```python
from build123d import *

# Parameters (mm, degrees)
SKETCH1_W           = 100
SKETCH1_H           = 100
BOSS_EXTRUDE1_DEPTH = 100
CUT_EXTRUDE16_DEPTH = 70
SKETCH8_W           = 70
SKETCH8_H           = 70
CUT_EXTRUDE17_DEPTH = 30
SKETCH9_W           = 21
SKETCH9_H           = 21
CUT_EXTRUDE20_DEPTH = 90
SKETCH10_W          = 30
SKETCH10_H          = 30
SKETCH10_W_2        = 16
SKETCH10_H_2        = 16
CUT_EXTRUDE21_DEPTH = 50
SKETCH11_W          = 30
SKETCH11_H          = 30
SKETCH11_W_2        = 20
SKETCH11_H_2        = 20
CUT_EXTRUDE22_DEPTH = 20
SKETCH12_W          = 30
SKETCH12_H          = 30
SKETCH12_W_2        = 20
SKETCH12_H_2        = 20
CUT_EXTRUDE23_DEPTH = 70
SKETCH13_W          = 20
SKETCH13_H          = 20
SKETCH13_W_2        = 16
SKETCH13_H_2        = 16
CUT_EXTRUDE24_DEPTH = 50
SKETCH15_R          = 2
CUT_EXTRUDE25_DEPTH = 30
SKETCH16_R          = 2
CUT_EXTRUDE26_DEPTH = 30
SKETCH17_R          = 2
CUT_EXTRUDE27_DEPTH = 16
SKETCH18_R          = 2
CUT_EXTRUDE29_DEPTH = 16
SKETCH19_W          = 30
SKETCH19_H          = 30
CUT_EXTRUDE30_DEPTH = 5
BOSS_EXTRUDE2_DEPTH = 20
SKETCH21_W          = 20
SKETCH21_H          = 7
BOSS_EXTRUDE6_DEPTH = 24
SKETCH22_W          = 2.5
SKETCH22_H          = 2.5
CUT_EXTRUDE31_DEPTH = 20
SKETCH23_W          = 7
SKETCH23_H          = 20
BOSS_EXTRUDE7_DEPTH = 24


with BuildPart() as part:
    # Sketch1 → Boss-Extrude1 (new body)
    with BuildSketch(Plane.XY):
        Rectangle(SKETCH1_W, SKETCH1_H)
    extrude(amount=-BOSS_EXTRUDE1_DEPTH)

    # Sketch5 → Cut-Extrude16 (cut)
    with BuildSketch(Plane(origin=(0, 0, -100), x_dir=(-1, 0, 0), z_dir=(0, 0, -1))):
        Polygon((50, -50), (50, 50), (-50, 50), (-50, -20), (-20, -20), (-20, -50), align=None)
    extrude(amount=-CUT_EXTRUDE16_DEPTH, mode=Mode.SUBTRACT)

    # Sketch8 → Cut-Extrude17 (cut)
    with BuildSketch(Plane(origin=(0, 0, -30), x_dir=(-1, 0, 0), z_dir=(0, 0, -1))):
        with Locations((15, 15)):
            Rectangle(SKETCH8_W, SKETCH8_H)
    extrude(amount=-CUT_EXTRUDE17_DEPTH, mode=Mode.SUBTRACT)

    # Sketch9 → Cut-Extrude20 (cut)
    with BuildSketch(Plane(origin=(0, 0, -100), x_dir=(-1, 0, 0), z_dir=(0, 0, -1))):
        with Locations((-35, -35)):
            Rectangle(SKETCH9_W, SKETCH9_H)
    extrude(amount=-CUT_EXTRUDE20_DEPTH, mode=Mode.SUBTRACT)

    # Sketch10 → Cut-Extrude21 (cut)
    with BuildSketch(Plane.ZY.offset(50)):
        with Locations((-15, -35)):
            Rectangle(SKETCH10_W, SKETCH10_H)
        with Locations((-15, -35)):
            Rectangle(SKETCH10_W_2, SKETCH10_H_2, mode=Mode.SUBTRACT)
    extrude(amount=-CUT_EXTRUDE21_DEPTH, mode=Mode.SUBTRACT)

    # Sketch11 → Cut-Extrude22 (cut)
    with BuildSketch(Plane.ZY):
        with Locations((-15, -35)):
            Rectangle(SKETCH11_W, SKETCH11_H)
        with Locations((-15, -35)):
            Rectangle(SKETCH11_W_2, SKETCH11_H_2, mode=Mode.SUBTRACT)
    extrude(amount=-CUT_EXTRUDE22_DEPTH, mode=Mode.SUBTRACT)

    # Sketch12 → Cut-Extrude23 (cut)
    with BuildSketch(Plane(origin=(0, 50, 0), x_dir=(1, 0, 0), z_dir=(0, 1, 0))):
        with Locations((35, 15)):
            Rectangle(SKETCH12_W, SKETCH12_H)
        with Locations((35, 15)):
            Rectangle(SKETCH12_W_2, SKETCH12_H_2, mode=Mode.SUBTRACT)
    extrude(amount=-CUT_EXTRUDE23_DEPTH, mode=Mode.SUBTRACT)

    # Sketch13 → Cut-Extrude24 (cut)
    with BuildSketch(Plane(origin=(0, 50, 0), x_dir=(1, 0, 0), z_dir=(0, 1, 0))):
        with Locations((35, 15)):
            Rectangle(SKETCH13_W, SKETCH13_H)
        with Locations((35, 15)):
            Rectangle(SKETCH13_W_2, SKETCH13_H_2, mode=Mode.SUBTRACT)
    extrude(amount=-CUT_EXTRUDE24_DEPTH, mode=Mode.SUBTRACT)

    # Sketch15 → Cut-Extrude25 (cut)
    with BuildSketch(Plane(origin=(0, -20, 0), x_dir=(1, 0, 0), z_dir=(0, 1, 0))):
        with Locations(Location((35, 85, 0), (0, 0, 270))):
            Circle(SKETCH15_R)
        with Locations(Location((35, 45, 0), (0, 0, 270))):
            Circle(SKETCH15_R)
    extrude(amount=-CUT_EXTRUDE25_DEPTH, mode=Mode.SUBTRACT)

    # Sketch16 → Cut-Extrude26 (cut)
    with BuildSketch(Plane(origin=(50, 0, 0), x_dir=(0, 0, -1), z_dir=(1, 0, 0))):
        with Locations((75, -35)):
            Circle(SKETCH16_R)
        with Locations((35, -35)):
            Circle(SKETCH16_R)
    extrude(amount=-CUT_EXTRUDE26_DEPTH, mode=Mode.SUBTRACT)

    # Sketch17 → Cut-Extrude27 (cut)
    with BuildSketch(Plane(origin=(0, 0, -23), x_dir=(-1, 0, 0), z_dir=(0, 0, -1))):
        with Locations((-35, 30)):
            Circle(SKETCH17_R)
        with Locations((-35, 10)):
            Circle(SKETCH17_R)
    extrude(amount=-CUT_EXTRUDE27_DEPTH, mode=Mode.SUBTRACT)

    # Sketch18 → Cut-Extrude29 (cut)
    with BuildSketch(Plane(origin=(0, 0, -23), x_dir=(-1, 0, 0), z_dir=(0, 0, -1))):
        with Locations((30, -35)):
            Circle(SKETCH18_R)
        with Locations((10, -35)):
            Circle(SKETCH18_R)
    extrude(amount=-CUT_EXTRUDE29_DEPTH, mode=Mode.SUBTRACT)

    # Sketch19 → Cut-Extrude30 (cut)
    with BuildSketch(Plane.XY):
        with Locations((35, -35)):
            Rectangle(SKETCH19_W, SKETCH19_H)
    extrude(amount=-CUT_EXTRUDE30_DEPTH, mode=Mode.SUBTRACT)

    # Sketch20 → Boss-Extrude2 (add)
    with BuildSketch(Plane.XY.offset(-5)):
        Polygon((25, 0), (0, -25), (0, -27), (27, -27), (27, 0), align=None)
    extrude(amount=-BOSS_EXTRUDE2_DEPTH)

    # Sketch21 → Boss-Extrude6 (add)
    with BuildSketch(Plane.ZY):
        with Locations((-15, -46.5)):
            Rectangle(SKETCH21_W, SKETCH21_H)
    extrude(amount=-BOSS_EXTRUDE6_DEPTH)

    # Sketch22 → Cut-Extrude31 (cut)
    with BuildSketch(Plane(origin=(0, 0, -25), x_dir=(-1, 0, 0), z_dir=(0, 0, -1))):
        with Locations((-25.75, -25.75)):
            Rectangle(SKETCH22_W, SKETCH22_H)
    extrude(amount=-CUT_EXTRUDE31_DEPTH, mode=Mode.SUBTRACT)

    # Sketch23 → Boss-Extrude7 (add)
    with BuildSketch(Plane(origin=(0, 0, 0), x_dir=(1, 0, 0), z_dir=(0, 1, 0))):
        with Locations((46.5, 15)):
            Rectangle(SKETCH23_W, SKETCH23_H)
    extrude(amount=-BOSS_EXTRUDE7_DEPTH)


solid = part.part
```
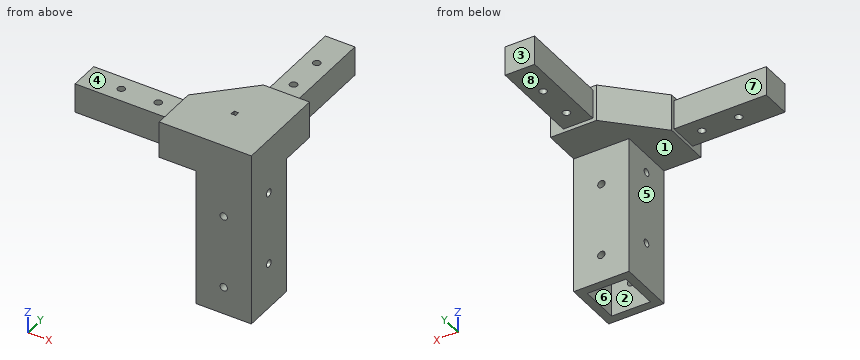
Verification items for the finished model (mm, model axes). Face numbers are marked on the shaded views. A direction names the side the tool comes from. Coordinates: 2 decimals unless noted, no trailing zeros. Order: outer loops, then holes, each group sorted by start corner. A loop starts at its lowest first (then second) coordinate and runs counter-clockwise, first axis right, second up. Notation, with made-up numbers: (33.25, 68.25) -> (71.25, 68.25) arc R33 ccw to (71.25, 100.25) -> close; hole circle Ø9 at (-8, -39.75). An arc over 180 degrees is marked (long way). Answer as CSV lines item,"result". Start each with the question number.
1) Cross-section at D-D, the plane x = -30. Record the boundary of the cut face in (y, z).
2) Set-up check for the marked faces 4, 5, 6, 7 and 8: record each of +Z, -Z, +X, -X, +Y, -Y from which the full face is reachable in a straight line by a thin tool's end or side.
3) Gauge pin test, flat ends, axial feed: pin 1 Ø13 at (y, z) = (13, -17.5) entering from -X; pin 2 Ø17 at (y, z) = (-38.5, -77) entering from -X; pin 3 Ø10 at (x, y) = (37.5, -14.5) entering from -Z. Record the tip position at first contact, or that the pin passes through.
4) Cross-section at C-C, the plane y = 30. Record the boundary of the cut face in (x, z).
5) Cross-section at B-B, the plane z = -67.5. Record the boundary of the cut face in (x, y), then the cut area to 3 significant figures.
6) Release check for a two-part mould opening along Y. For the marked faces 1, 2 and 3 record: released by +Y, released by -Y, zero draft, split by the parting line, or undercut.
7) Cross-section at A-A, the plane z = -85. Record the boundary of the cut face in (x, y).
8) Material ranges on L1, parallel to X at y = -40, z = -38; L2, parallel to Y at x = 39, z = -92; L3, parallel to Y at x = -10, z = -12.5, recorded low to high. Write a range as [from, to].
Conclusion:
1,outline,"(-43, -23) -> (-37, -23) -> (-37, -7) -> (-43, -7) -> close; (-33, -23) -> (-27, -23) -> (-27, -7) -> (-33, -7) -> close"
2,face 4,"+Z, -X, +Y, -Y"
2,face 5,"-Z, -X, +Y, -Y"
2,face 6,"-Z"
2,face 7,"+Z, -Z, -X, +Y"
2,face 8,"-Z, +X, -X, +Y"
3,pin 1,"stops at x = 27"
3,pin 2,"stops at x = 20"
3,pin 3,"stops at z = -25"
4,outline,"(27, -23) -> (33, -23) -> (33, -7) -> (27, -7) -> close; (37, -23) -> (43, -23) -> (43, -7) -> (37, -7) -> close"
5,outline,"(20, -50) -> (50, -50) -> (50, -20) -> (20, -20) -> close; hole (24.5, -45.5) -> (45.5, -45.5) -> (45.5, -24.5) -> (24.5, -24.5) -> close"
5,area,"459 mm²"
6,face 1,"zero draft"
6,face 2,"undercut"
6,face 3,"released by +Y"
7,outline,"(20, -50) -> (33, -50) -> (33, -45.5) -> (24.5, -45.5) -> (24.5, -24.5) -> (33, -24.5) -> (33, -20) -> (20, -20) -> close; (37, -50) -> (50, -50) -> (50, -20) -> (37, -20) -> (37, -24.5) -> (45.5, -24.5) -> (45.5, -45.5) -> (37, -45.5) -> close"
8,L1,"x = [20, 24.5], [45.5, 50]"
8,L2,"y = [-50, -45.5], [-24.5, -20]"
8,L3,"y = [-43, -37], [-33, -27]"
